Work out the finished part from the listing and answer in its coordinate system (mm). A direction names the side the tool comes from. Round coordinates to 2 decimals unless told otherwise and drop trailing zeros. Order: outer loops, then holes, each group sorted by start corner. A loop starts at its lowest first (then second) coordinate and runs counter-clockwise, first axis right, second up. Notation, with made-up numbers: (-6.75, -38.5) - (50.25, -38.5) arc R14 cw to (50.25, -17.5) - close; hole circle Ø7 at (-10.75, 10). An arc over 180 degrees is marked (long way). Use CSV: the item, a comma, the result in double quotes.
from build123d import *

# Parameters (mm, degrees)
SKETCH1_W                       = 165.1
SKETCH1_H                       = 142.875
BOSS_EXTRUDE1_DEPTH             = 12.7
BOSS_EXTRUDE2_DEPTH             = 12.7
CUT_EXTRUDE1_REACH              = 116.135
BOSS_EXTRUDE3_DEPTH             = 12.7
CUT_EXTRUDE2_DEPTH              = 12.7
F_21_0_159_DIAMETER_HOLE1_D     = 4.0386
F_21_0_159_DIAMETER_HOLE1_DEPTH = 22.225
F_21_0_159_DIAMETER_HOLE1_TIP   = 1.213317848
F_21_0_159_DIAMETER_HOLE2_D     = 4.0386
F_21_0_159_DIAMETER_HOLE2_DEPTH = 22.225
F_21_0_159_DIAMETER_HOLE2_TIP   = 1.213317848
SKETCH21_R                      = 4.7625
SKETCH21_R_2                    = 3.175
CUT_EXTRUDE10_DEPTH             = 6.35
F_8_CLEARANCE_HOLE1_D           = 4.4958
F_8_CLEARANCE_HOLE1_DEPTH       = 19.05
F_8_CLEARANCE_HOLE1_TIP         = 1.350674586
SKETCH24_W                      = 9.525
SKETCH24_H                      = 12.7
CUT_EXTRUDE11_DEPTH             = 115.134515622
FILLET1_R                       = 6.35
SKETCH29_W                      = 9.525
SKETCH29_H                      = 26.350000132
CUT_EXTRUDE12_DEPTH             = 6.35
FILLET2_R                       = 3.175
F_8_CLEARANCE_HOLE2_D           = 4.4958
SKETCH32_W                      = 7.9375
SKETCH32_H                      = 20.6375
CUT_EXTRUDE13_DEPTH             = 115.134515622
CUT_EXTRUDE14_START             = -6.35
CUT_EXTRUDE14_DEPTH             = 6.35
FILLET3_R                       = 3.175
CUT_EXTRUDE15_DEPTH             = 6.35
F_8_CLEARANCE_HOLE3_D           = 4.4958
CUT_EXTRUDE16_DEPTH             = 115.134515622
FILLET4_R                       = 2.54


with BuildPart() as part:
    # Sketch1 → Boss-Extrude1 (new body)
    with BuildSketch(Plane.XY):
        Rectangle(SKETCH1_W, SKETCH1_H)
    extrude(amount=BOSS_EXTRUDE1_DEPTH)

    # Sketch2 → Boss-Extrude2 (add)
    with BuildSketch(Plane.XY.offset(12.7)):
        Polygon((-11.1125, 71.4375), (11.1125, 71.4375), (11.1125, 75.2475), (10.664629469, 77.7875), (-10.664629469, 77.7875), (-11.1125, 75.2475), align=None)
    extrude(amount=-BOSS_EXTRUDE2_DEPTH)

    # Sketch4 → Cut-Extrude1 (cut, up to next)
    with BuildSketch(Plane.XY.offset(12.7), mode=Mode.PRIVATE) as cut_extrude1_sk1:
        with BuildLine():
            Line((-17.7165, 71.4375), (-11.1125, 71.4375))
            ThreePointArc((-11.1125, 71.4375), (-14.4145, 68.1355), (-17.7165, 71.4375))
        make_face()
    cut_extrude1_tool1 = extrude(cut_extrude1_sk1.sketch, amount=-CUT_EXTRUDE1_REACH, mode=Mode.PRIVATE) & part.part
    # Sketch4 → Cut-Extrude1 (cut, up to next)
    with BuildSketch(Plane.XY.offset(12.7), mode=Mode.PRIVATE) as cut_extrude1_sk2:
        with BuildLine():
            Line((11.1125, 71.4375), (17.7165, 71.4375))
            ThreePointArc((17.7165, 71.4375), (14.4145, 68.1355), (11.1125, 71.4375))
        make_face()
    cut_extrude1_tool2 = extrude(cut_extrude1_sk2.sketch, amount=-CUT_EXTRUDE1_REACH, mode=Mode.PRIVATE) & part.part
    add(cut_extrude1_tool1.solids().sort_by_distance((-14.4145, 70.036088, 12.7))[0], mode=Mode.SUBTRACT)
    add(cut_extrude1_tool2.solids().sort_by_distance((14.4145, 70.036088, 12.7))[0], mode=Mode.SUBTRACT)

    # Sketch5 → Boss-Extrude3 (add)
    with BuildSketch(Plane.XY.offset(12.7)):
        Polygon((50.8, -71.4375), (28.575, -71.4375), (28.575, -75.2475), (29.022870531, -77.7875), (50.352129469, -77.7875), (50.8, -75.2475), align=None)
    boss_extrude3 = extrude(amount=-BOSS_EXTRUDE3_DEPTH)

    # Sketch6 → Cut-Extrude2 (cut)
    with BuildSketch(Plane.XY.offset(12.7)):
        with BuildLine():
            Line((21.971, -71.4375), (28.575, -71.4375))
            ThreePointArc((28.575, -71.4375), (25.273, -68.1355), (21.971, -71.4375))
        make_face()
        with BuildLine():
            Line((50.8, -71.4375), (57.404, -71.4375))
            ThreePointArc((57.404, -71.4375), (54.102, -68.1355), (50.8, -71.4375))
        make_face()
    cut_extrude2 = extrude(amount=-CUT_EXTRUDE2_DEPTH, mode=Mode.SUBTRACT)

    # Mirror1: Boss-Extrude3, Cut-Extrude2 across plane
    add(boss_extrude3.mirror(Plane(origin=(0, 0, 0), x_dir=(0, 0, 1), z_dir=(1, 0, 0))))
    add(cut_extrude2.mirror(Plane(origin=(0, 0, 0), x_dir=(0, 0, 1), z_dir=(1, 0, 0))), mode=Mode.SUBTRACT)

    # #21 (0.159) Diameter Hole1
    with Locations(Plane(origin=(82.55, 0, 0), x_dir=(0, 0, -1), z_dir=(1, 0, 0))):
        with Locations((-6.35, 4.7625)):
            Hole(F_21_0_159_DIAMETER_HOLE1_D / 2, depth=F_21_0_159_DIAMETER_HOLE1_DEPTH)
            with Locations((0, 0, -(F_21_0_159_DIAMETER_HOLE1_DEPTH + F_21_0_159_DIAMETER_HOLE1_TIP / 2))):  # 118° drill point
                Cone(0, F_21_0_159_DIAMETER_HOLE1_D / 2, F_21_0_159_DIAMETER_HOLE1_TIP, mode=Mode.SUBTRACT)

    # #21 (0.159) Diameter Hole2
    with Locations(Plane.ZY.offset(82.55)):
        with Locations((6.35, 4.7625)):
            Hole(F_21_0_159_DIAMETER_HOLE2_D / 2, depth=F_21_0_159_DIAMETER_HOLE2_DEPTH)
            with Locations((0, 0, -(F_21_0_159_DIAMETER_HOLE2_DEPTH + F_21_0_159_DIAMETER_HOLE2_TIP / 2))):  # 118° drill point
                Cone(0, F_21_0_159_DIAMETER_HOLE2_D / 2, F_21_0_159_DIAMETER_HOLE2_TIP, mode=Mode.SUBTRACT)

    # Sketch21 → Cut-Extrude10 (cut)
    with BuildSketch(Plane(origin=(0, 0, 0), x_dir=(-1, 0, 0), z_dir=(0, 0, -1))):
        with Locations((-57.15, 36.5125)):
            Circle(SKETCH21_R)
        with Locations((57.15, 36.5125)):
            Circle(SKETCH21_R)
        with Locations((3.263048163, -2.752650538)):
            Circle(SKETCH21_R_2)
    extrude(amount=-CUT_EXTRUDE10_DEPTH, mode=Mode.SUBTRACT)

    # #8 Clearance Hole1
    with Locations(Plane(origin=(0, 0, 0), x_dir=(-1, 0, 0), z_dir=(0, 0, -1))):
        with Locations((-57.15, 36.5125), (3.263048163, -2.752650538), (57.15, 36.5125)):
            Hole(F_8_CLEARANCE_HOLE1_D / 2, depth=F_8_CLEARANCE_HOLE1_DEPTH)
            with Locations((0, 0, -(F_8_CLEARANCE_HOLE1_DEPTH + F_8_CLEARANCE_HOLE1_TIP / 2))):  # 118° drill point
                Cone(0, F_8_CLEARANCE_HOLE1_D / 2, F_8_CLEARANCE_HOLE1_TIP, mode=Mode.SUBTRACT)

    # Sketch24 → Cut-Extrude11 (cut, through all)
    with BuildSketch(Plane.XY.offset(12.7)):
        with Locations((-77.7875, -65.0875)):
            Rectangle(SKETCH24_W, SKETCH24_H)
        with Locations((77.7875, -65.0875)):
            Rectangle(SKETCH24_W, SKETCH24_H)
    extrude(amount=-CUT_EXTRUDE11_DEPTH, mode=Mode.SUBTRACT)

    # Fillet1
    fillet1_edges = [part.edges().sort_by_distance(p)[0] for p in [
        (-73.025, -58.7375, 6.35),
        (73.025, -58.7375, 6.35),
    ]]
    fillet(fillet1_edges, radius=FILLET1_R)

    # Sketch29 → Cut-Extrude12 (cut)
    with BuildSketch(Plane(origin=(0, 0, 0), x_dir=(-1, 0, 0), z_dir=(0, 0, -1))):
        with Locations((62.70625, 58.262499934)):
            Rectangle(SKETCH29_W, SKETCH29_H)
    extrude(amount=-CUT_EXTRUDE12_DEPTH, mode=Mode.SUBTRACT)

    # Fillet2
    fillet2_edges = [part.edges().sort_by_distance(p)[0] for p in [
        (-57.94375, 45.087499868, 3.175),
        (-67.46875, 45.087499868, 3.175),
    ]]
    fillet(fillet2_edges, radius=FILLET2_R)

    # #8 Clearance Hole2 (through all)
    with Locations(Plane(origin=(0, 0, 6.35), x_dir=(-1, 0, 0), z_dir=(0, 0, -1))):
        with Locations((62.70625, 64.612499934), (62.70625, 51.912499934)):
            Hole(F_8_CLEARANCE_HOLE2_D / 2)

    # Sketch32 → Cut-Extrude13 (cut, through all)
    with BuildSketch(Plane(origin=(0, 0, 0), x_dir=(-1, 0, 0), z_dir=(0, 0, -1))):
        with Locations((71.4375, 58.262499934)):
            Rectangle(SKETCH32_W, SKETCH32_H)
    extrude(amount=-CUT_EXTRUDE13_DEPTH, mode=Mode.SUBTRACT)

    # Sketch33 → Cut-Extrude14 (cut)
    with BuildSketch(Plane(origin=(0, 0, 0), x_dir=(-1, 0, 0), z_dir=(0, 0, -1)).offset(CUT_EXTRUDE14_START)):
        with BuildLine():
            Line((67.46875, 47.943749934), (67.45270924, 47.943749934))
            ThreePointArc((67.45270924, 47.943749934), (67.464737274, 48.10292322), (67.46875, 48.262499868))
            Line((67.46875, 48.262499868), (67.46875, 47.943749934))
        make_face()
    extrude(amount=CUT_EXTRUDE14_DEPTH, mode=Mode.SUBTRACT)

    # Fillet3
    fillet3_edges = [part.edges().sort_by_distance(p)[0] for p in [
        (-67.46875, 47.943749934, 9.525),
        (-67.46875, 68.581249934, 9.525),
        (-75.40625, 68.581249934, 6.35),
        (-75.40625, 47.943749934, 6.35),
    ]]
    fillet(fillet3_edges, radius=FILLET3_R)

    # Sketch34 → Cut-Extrude15 (cut)
    with BuildSketch(Plane(origin=(0, 0, 0), x_dir=(-1, 0, 0), z_dir=(0, 0, -1))):
        Polygon((40.757720371, 5.302804118), (53.841519997, 28.906603465), (62.172272708, 24.288791832), (49.088473081, 0.684992485), align=None)
    extrude(amount=-CUT_EXTRUDE15_DEPTH, mode=Mode.SUBTRACT)

    # #8 Clearance Hole3 (through all)
    with Locations(Plane(origin=(0, 0, 6.35), x_dir=(-1, 0, 0), z_dir=(0, 0, -1))):
        with Locations((54.543537628, 20.349633115), (48.386455451, 9.241962835)):
            Hole(F_8_CLEARANCE_HOLE3_D / 2)

    # Sketch37 → Cut-Extrude16 (cut, through all)
    with BuildSketch(Plane(origin=(0, 0, 0), x_dir=(-1, 0, 0), z_dir=(0, 0, -1))):
        Polygon((60.633002164, 21.511874262), (67.575296089, 17.663697901), (57.570037551, -0.386266305), (50.627743626, 3.461910055), align=None)
    extrude(amount=-CUT_EXTRUDE16_DEPTH, mode=Mode.SUBTRACT)

    # Fillet4
    fillet4_edges = [part.edges().sort_by_distance(p)[0] for p in [
        (-49.088473081, 0.684992485, 3.175),
        (-40.757720371, 5.302804118, 3.175),
        (-53.841519997, 28.906603465, 3.175),
        (-62.172272708, 24.288791832, 3.175),
        (-67.575296089, 17.663697901, 6.35),
        (-50.627743626, 3.461910055, 9.525),
        (-57.570037551, -0.386266305, 6.35),
        (-60.633002164, 21.511874262, 9.525),
    ]]
    fillet(fillet4_edges, radius=FILLET4_R)


solid = part.part
(1) Each of these flat-tipped pins is pushed along its axis until it touches: pin 1 (3.5 mm diameter, centred on y = 4.76, z = 6.35, fed in from +X); pin 2 (7 mm diameter, centred on x = -57.15, y = 36.51, fed in from +Z); pin 3 (2.5 mm diameter, centred on x = 81, z = 8, fed in from -Y); pin 4 (3 mm diameter, centred on y = 4.76, z = 6.35, fed in from +X). Where does it stop, or does it pass through?
Findings below:
pin 1,"stops at x = 60.16"
pin 2,"stops at z = 12.7"
pin 3,"stops at y = -58.74"
pin 4,"stops at x = 60.01"
(2) Find section A-A (x = -38). Determine the outline of the cut face in (y, z), and give its area (3 significant figures).
Findings below:
outline,"(-77.79, 0) - (71.44, 0) - (71.44, 12.7) - (-77.79, 12.7) - close"
area,"1,900 mm²"
(3) For faces 3 (the flat face through (73.025, -68, 6)), 4 (the flat face through (11.112, 73, 6)), 5 (the flat face through (-44.95, 2.98, 3.13)), 6 (the flat face through (-62.625, 8.734, 6.261)), 7 (the flat face through (-50.8, -73, 6)), determine the directions among +Z, -Z, +X, -X, +Y, -Y from which every point of the face is accessible in a straight line to the end or side of a thin tool.
Findings below:
face 3,"+Z, -Z, +X, -Y"
face 4,"+Z, -Z, +X, +Y"
face 5,"-Z"
face 6,"+Z, -Z"
face 7,"+Z, -Z, -X, -Y"
(4) Find the intervals of material crossed by L1, parallel to X at y = 63, z = 10.75; L2, parallel to X at y = 40, z = 1.5; L3, parallel to Y at x = -74.5, z = 7, in increasing order. Write a range as from..to.
Findings below:
L1,"x = -82.55..-75.41, -67.47..-64.27, -61.14..82.55"
L2,"x = -82.55..-60.39, -53.91..53.91, 60.39..82.55"
L3,"y = -61.02..2.85, 6.67..48.9, 67.63..71.44"
(5) Find section B-B (x = 15.5). Determine the outline of the cut face in (y, z), and give its area (3 significant figures).
Findings below:
outline,"(-71.44, 0) - (68.32, 0) - (68.32, 12.7) - (-71.44, 12.7) - close"
area,"1,770 mm²"
(6) The mould has two halves that part along Z. Classify faces 1 (the cylindrical face through (-71.28, 2.97, 5.42)), 2 (the flat face through (-11.112, 73, 6)): released by +Z, released by -Z, zero draft, split by the parting line, or undercut.
Findings below:
face 1,"undercut"
face 2,"zero draft"
